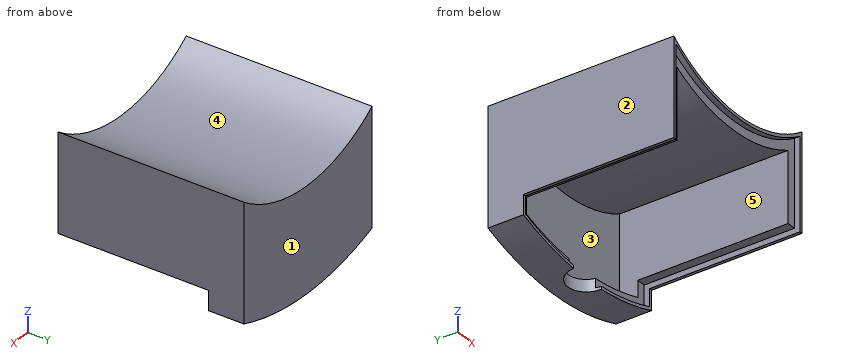
```python
from build123d import *

# Parameters (mm, degrees)
BOSS_EXTRUDE2_DEPTH  = 2
BOSS_EXTRUDE9_DEPTH  = 3
BOSS_EXTRUDE10_DEPTH = 0.9
SKETCH20_R           = 3.25
CUT_EXTRUDE14_DEPTH  = 20.9
SKETCH21_W           = 30
SKETCH21_H           = 16.85185618
CUT_EXTRUDE15_DEPTH  = 1
BOSS_EXTRUDE11_DEPTH = 25
SKETCH23_W           = 0.5
SKETCH23_H           = 24.1
BOSS_EXTRUDE12_DEPTH = 0.9
BOSS_EXTRUDE13_DEPTH = 0.9


with BuildPart() as part:
    # Sketch1 → Boss-Extrude2 (new body)
    with BuildSketch(Plane(origin=(0, 0, 0), x_dir=(1, 0, 0), z_dir=(0, 1, 0))):
        with BuildLine():
            Line((-15, 39.764934301), (-15, 20.264934301))
            ThreePointArc((-15, 20.264934301), (0, 25.212448557), (15, 20.264934301))
            Line((15, 20.264934301), (15, 39.764934301))
            ThreePointArc((15, 39.764934301), (0, 42.5), (-15, 39.764934301))
        make_face()
    extrude(amount=BOSS_EXTRUDE2_DEPTH)

    # Sketch16 → Boss-Extrude9 (add)
    with BuildSketch(Plane.XZ):
        with BuildLine():
            Line((-15, -20.264934301), (-15, -39.764934301))
            ThreePointArc((-15, -39.764934301), (0, -42.5), (15, -39.764934301))
            Line((15, -39.764934301), (15, -20.264934301))
            ThreePointArc((15, -20.264934301), (0, -25.212448557), (-15, -20.264934301))
        make_face()
        with BuildLine():
            ThreePointArc((-13, -38.356876828), (0, -40.5), (13, -38.356876828))
            Line((13, -38.356876828), (13, -23.906429187))
            ThreePointArc((13, -23.906429187), (0, -27.212448557), (-13, -23.906429187))
            Line((-13, -23.906429187), (-13, -38.356876828))
        make_face(mode=Mode.SUBTRACT)
    extrude(amount=BOSS_EXTRUDE9_DEPTH)

    # Sketch17 → Boss-Extrude10 (add)
    with BuildSketch(Plane.XZ.offset(3)):
        with BuildLine():
            ThreePointArc((15, -20.264934301), (0, -25.212448557), (-15, -20.264934301))
            Line((-15, -20.264934301), (-15, -39.764934301))
            ThreePointArc((-15, -39.764934301), (0, -42.5), (15, -39.764934301))
            Line((15, -39.764934301), (15, -20.264934301))
        make_face()
        with BuildLine():
            ThreePointArc((-14.5, -39.417635647), (0, -42), (14.5, -39.417635647))
            Line((14.5, -39.417635647), (14.5, -21.233935358))
            ThreePointArc((14.5, -21.233935358), (0, -25.712448557), (-14.5, -21.233935358))
            Line((-14.5, -21.233935358), (-14.5, -39.417635647))
        make_face(mode=Mode.SUBTRACT)
    extrude(amount=BOSS_EXTRUDE10_DEPTH)

    # Sketch20 → Cut-Extrude14 (cut)
    with BuildSketch(Plane.XY.offset(-50)):
        with Locations((0, -3.9)):
            Circle(SKETCH20_R)
    extrude(amount=CUT_EXTRUDE14_DEPTH, mode=Mode.SUBTRACT)

    # Sketch21 → Cut-Extrude15 (cut)
    with BuildSketch(Plane.XZ.offset(3)):
        with Locations((0, -27.189006211)):
            Rectangle(SKETCH21_W, SKETCH21_H)
    extrude(amount=CUT_EXTRUDE15_DEPTH, mode=Mode.SUBTRACT)

    # Sketch22 → Boss-Extrude11 (add)
    with BuildSketch(Plane.XZ.offset(3)):
        with BuildLine():
            Line((15, -20.264934301), (15, -35.614934301))
            Line((15, -35.614934301), (13, -35.614934301))
            Line((13, -35.614934301), (13, -23.906429187))
            ThreePointArc((13, -23.906429187), (0, -27.212448557), (-13, -23.906429187))
            Line((-13, -23.906429187), (-13, -35.614934301))
            Line((-13, -35.614934301), (-15, -35.614934301))
            Line((-15, -35.614934301), (-15, -20.264934301))
            ThreePointArc((-15, -20.264934301), (0, -25.212448557), (15, -20.264934301))
        make_face()
    extrude(amount=BOSS_EXTRUDE11_DEPTH)

    # Sketch23 → Boss-Extrude12 (add)
    with BuildSketch(Plane(origin=(0, 0, -35.614934301), x_dir=(-1, 0, 0), z_dir=(0, 0, -1))):
        with Locations((-14.75, -15.95)):
            Rectangle(SKETCH23_W, SKETCH23_H)
        with Locations((14.75, -15.95)):
            Rectangle(SKETCH23_W, SKETCH23_H)
    extrude(amount=BOSS_EXTRUDE12_DEPTH)

    # Sketch26 → Boss-Extrude13 (add)
    with BuildSketch(Plane.XZ.offset(28)):
        with BuildLine():
            Line((15, -36.514934301), (15, -20.264934301))
            ThreePointArc((15, -20.264934301), (0, -25.212448557), (-15, -20.264934301))
            Line((-15, -20.264934301), (-15, -36.514934301))
            Line((-15, -36.514934301), (-14.5, -36.514934301))
            Line((-14.5, -36.514934301), (-14.5, -21.233935358))
            ThreePointArc((-14.5, -21.233935358), (0, -25.712448557), (14.5, -21.233935358))
            Line((14.5, -21.233935358), (14.5, -36.514934301))
            Line((14.5, -36.514934301), (15, -36.514934301))
        make_face()
    extrude(amount=BOSS_EXTRUDE13_DEPTH)


solid = part.part
```
CAD build for the part. Positions are in the model's coordinates, mm. Face numbers are marked on the shaded views. A direction names the side the tool comes from. Coordinates: 2 decimals unless noted, no trailing zeros. Write each loop counter-clockwise with the first axis right and the second up, starting at its lowest first coordinate (ties: lowest second). Pieces come first, ordered by that corner, then holes.
(1) Two-plate mould, pull along X, no slides. Class the marked faces 1, 2 and 3: +X half, -X half, draft (parallel to the pull), parting line (faces both ways), or undercut.
(2) Cut at C-C, the plane z = -24.5. List the corners of the cut face in (x, y).
(3) Cut at B-B, the plane x = 0. List the corners of the cut face in (y, z).
(4) Cut at D-D, the plane y = -17. List the corners of the cut face in (x, z), and give its area (3 significant figures).
(5) Cut at A-A, the plane z = -34.25. List the corners of the cut face in (x, y), and give its area (3 significant figures).
(6) Drill centre lines: probe 1 along X at (y, z) = (-4.5, -30.5); probe 2 along Y at (x, z) = (12, -32.25); probe 3 along Y at (x, z) = (13.5, -33). Where is each one in solid material? Low to high.
(7) Flat gauge pins, fed straight in: pin 1 (3 mm diameter, centred on x = -7, y = -8, fed in from -Z); pin 2 (1.6 mm diameter, centred on x = 13.5, y = -18.5, fed in from -Z); pin 3 (12 mm diameter, centred on x = 1, y = -18, fed in from +Z). Where does each tip first touch, or does it go through?
(8) 3-axis set-ups, long thin cutter, end or side, ignore diameter. For the marked faces 4 and 5: which of +Z, -Z, +X, -X, +Y, -Y reach the whole face in a straight line?
Geometry says:
1. face 1: draft
1. face 2: -X half
1. face 3: undercut
2. outline: (-15, -28.9) - (-14.5, -28.9) - (-14.5, -28) - (-13, -28) - (-13, 0) - (-11.84, 0) - (-11.84, -28) - (-7.8, -28) - (-7.8, -28.9) - (-5.95, -28.9) - (-5.95, 2) - (-15, 2) - close; (5.95, -28.9) - (7.8, -28.9) - (7.8, -28) - (11.84, -28) - (11.84, 0) - (13, 0) - (13, -28) - (14.5, -28) - (14.5, -28.9) - (15, -28.9) - (15, 2) - (5.95, 2) - close
3. outline: (-28.9, -25.71) - (-28, -25.71) - (-28, -27.21) - (0, -27.21) - (0, -40.5) - (-0.65, -40.5) - (-0.65, -42.5) - (2, -42.5) - (2, -25.21) - (-28.9, -25.21) - close
4. outline: (-15, -36.51) - (-14.5, -36.51) - (-14.5, -35.61) - (-13, -35.61) - (-13, -23.91) arc R27.21 ccw to (13, -23.91) - (13, -35.61) - (14.5, -35.61) - (14.5, -36.51) - (15, -36.51) - (15, -20.26) arc R25.21 cw to (-15, -20.26) - close
4. area: 114 mm2
5. outline: (-15, -28.9) - (-14.5, -28.9) - (-14.5, -28) - (-13, -28) - (-13, 0) - (13, 0) - (13, -28) - (14.5, -28) - (14.5, -28.9) - (15, -28.9) - (15, 2) - (-15, 2) - close
5. area: 173 mm2
6. probe 1: x = -15 to -13, 13 to 15
6. probe 2: y = 0 to 2
6. probe 3: y = -28 to 2
7. pin 1: stops at z = -26.65
7. pin 2: stops at z = -35.61
7. pin 3: stops at z = -24.22
8. face 4: +Z, +Y, -Y
8. face 5: -Y
